Can you work these out from the model? Positions are in its coordinate system, mm. A direction names the side the tool comes from. Round coordinates to 2 decimals unless told otherwise and drop trailing zeros. Loops run counter-clockwise (first coordinate to the right, second up) from the corner with the lowest first, then second, coordinate; pieces in that order, holes last. Notation, with made-up numbers: (-21.75, 82) -> (-9.75, 82) arc R16 cw to (-9.75, 92) -> close; hole circle Ø3 at (87.25, 25). An arc over 180 degrees is marked (long way). Use a Markdown table: item, result.
from build123d import *

# Parameters (mm, degrees)
ESBO_O1_W                  = 50
ESBO_O1_H                  = 600
RESSALTO_EXTRUS_O1_DEPTH   = 200
ESBO_O1_W_2                = 47.772216991
RESSALTO_EXTRUS_O1_2_DEPTH = 200
RESSALTO_EXTRUS_O4_START   = -210
ESBO_O4_W                  = 600
ESBO_O4_H                  = 600
RESSALTO_EXTRUS_O4_DEPTH   = 10
ESBO_O5_W                  = 200
ESBO_O5_H                  = 190
CORTE_EXTRUS_O1_DEPTH      = 872.779788708
ESBO_O6_W                  = 200
ESBO_O6_H                  = 190
CORTE_EXTRUS_O2_DEPTH      = 600
FILETE2_R                  = 20
FILETE3_SIZE               = 20
FILETE4_SIZE               = 20
FILETE5_SIZE               = 20


with BuildPart() as part:
    # Esbo_o1 → Ressalto-extrus_o1 (new body)
    with BuildSketch(Plane(origin=(0, 0, 0), x_dir=(1, 0, 0), z_dir=(0, 1, 0))):
        with Locations((25, 300)):
            Rectangle(ESBO_O1_W, ESBO_O1_H)
    extrude(amount=RESSALTO_EXTRUS_O1_DEPTH)



with BuildPart() as body_2:
    # Esbo_o1 → Ressalto-extrus_o1 2 (new body)
    with BuildSketch(Plane(origin=(0, 0, 0), x_dir=(1, 0, 0), z_dir=(0, 1, 0))):
        with Locations((576.113891505, 300)):
            Rectangle(ESBO_O1_W_2, ESBO_O1_H)
    extrude(amount=RESSALTO_EXTRUS_O1_2_DEPTH)


with BuildPart() as part_1:
    add(part.part)

    add(body_2.part)  # Ressalto-extrus_o4 merges body 2
    # Esbo_o4 → Ressalto-extrus_o4 (add)
    with BuildSketch(Plane(origin=(0, 200, 0), x_dir=(1, 0, 0), z_dir=(0, 1, 0)).offset(RESSALTO_EXTRUS_O4_START)):
        with Locations((300, 300)):
            Rectangle(ESBO_O4_W, ESBO_O4_H)
    extrude(amount=RESSALTO_EXTRUS_O4_DEPTH)

    # Esbo_o5 → Corte-extrus_o1 (cut, through all)
    with BuildSketch(Plane(origin=(600, 0, 0), x_dir=(0, 0, -1), z_dir=(1, 0, 0))):
        with Locations((100, 105)):
            Rectangle(ESBO_O5_W, ESBO_O5_H)
    extrude(amount=-CORTE_EXTRUS_O1_DEPTH, mode=Mode.SUBTRACT)

    # Esbo_o6 → Corte-extrus_o2 (cut)
    with BuildSketch(Plane(origin=(600, 0, 0), x_dir=(0, 0, -1), z_dir=(1, 0, 0))):
        with Locations((500, 105)):
            Rectangle(ESBO_O6_W, ESBO_O6_H)
    extrude(amount=-CORTE_EXTRUS_O2_DEPTH, mode=Mode.SUBTRACT)

    # Filete2
    filete2_edges = [part_1.edges().sort_by_distance(p)[0] for p in [
        (576.113891505, 200, -200),
    ]]
    fillet(filete2_edges, radius=FILETE2_R)

    # Filete3
    # a fillet whose section is not a circle: 20 mm, written as the material it takes off along each edge
    with BuildSketch(Plane(origin=(650, 200, -400), x_dir=(0, 0, 1), z_dir=(-1, 0, 0))) as filete3_piece_1:
        with BuildLine():
            add(Edge.make_bspline([(FILETE3_SIZE, 0), (FILETE3_SIZE * 0.831801948466, 0), (FILETE3_SIZE * 0.663603896932, 0), (FILETE3_SIZE * 0.292893218813, -FILETE3_SIZE * 0.0716919198361), (FILETE3_SIZE * 0.0716919198361, -FILETE3_SIZE * 0.292893218813), (0, -FILETE3_SIZE * 0.663603896932), (0, -FILETE3_SIZE * 0.831801948466), (0, -FILETE3_SIZE)], knots=[0, 0, 0, 0, 0, 0, 0.5, 0.5, 1, 1, 1, 1, 1, 1], degree=5))
            Line((0, -FILETE3_SIZE), (0, 0))
            Line((0, 0), (FILETE3_SIZE, 0))
        make_face()
    extrude(amount=147.772216991, mode=Mode.SUBTRACT)

    # Filete4
    # a fillet whose section is not a circle: 20 mm, written as the material it takes off along each edge
    with BuildSketch(Plane(origin=(100, 200, -200), x_dir=(0, -1, 0), z_dir=(-1, 0, 0))) as filete4_piece_1:
        with BuildLine():
            add(Edge.make_bspline([(FILETE4_SIZE, 0), (FILETE4_SIZE * 0.831801948466, 0), (FILETE4_SIZE * 0.663603896932, 0), (FILETE4_SIZE * 0.292893218813, -FILETE4_SIZE * 0.0716919198361), (FILETE4_SIZE * 0.0716919198361, -FILETE4_SIZE * 0.292893218813), (0, -FILETE4_SIZE * 0.663603896932), (0, -FILETE4_SIZE * 0.831801948466), (0, -FILETE4_SIZE)], knots=[0, 0, 0, 0, 0, 0, 0.5, 0.5, 1, 1, 1, 1, 1, 1], degree=5))
            Line((0, -FILETE4_SIZE), (0, 0))
            Line((0, 0), (FILETE4_SIZE, 0))
        make_face()
    extrude(amount=150, mode=Mode.SUBTRACT)

    # Filete5
    # a fillet whose section is not a circle: 20 mm, written as the material it takes off along each edge
    with BuildSketch(Plane(origin=(100, 200, -400), x_dir=(0, 0, 1), z_dir=(-1, 0, 0))) as filete5_piece_1:
        with BuildLine():
            add(Edge.make_bspline([(FILETE5_SIZE, 0), (FILETE5_SIZE * 0.831801948466, 0), (FILETE5_SIZE * 0.663603896932, 0), (FILETE5_SIZE * 0.292893218813, -FILETE5_SIZE * 0.0716919198361), (FILETE5_SIZE * 0.0716919198361, -FILETE5_SIZE * 0.292893218813), (0, -FILETE5_SIZE * 0.663603896932), (0, -FILETE5_SIZE * 0.831801948466), (0, -FILETE5_SIZE)], knots=[0, 0, 0, 0, 0, 0, 0.5, 0.5, 1, 1, 1, 1, 1, 1], degree=5))
            Line((0, -FILETE5_SIZE), (0, 0))
            Line((0, 0), (FILETE5_SIZE, 0))
        make_face()
    extrude(amount=150, mode=Mode.SUBTRACT)


solid = part_1.part
1. I want a section at B-B (z = -491). Please give me the cut outline in (x, y), plus the area to 3 significant figures.
Answer sheet:
| item | result |
|---|---|
| outline | (0, -10) -> (600, -10) -> (600, 10) -> (552.23, 10) -> (552.23, 0) -> (50, 0) -> (50, 10) -> (0, 10) -> close |
| area | 6,980 mm² |
2. Will these pins go through, and if not, where does the flat tip stop? pin 1 Ø14.5 at (x, y) = (570, 114.5) entering from -Z; pin 2 Ø3 at (x, z) = (424.5, -315) entering from +Y; pin 3 Ø14.5 at (x, z) = (582.5, -52.5) entering from +Y.
Answer sheet:
| item | result |
|---|---|
| pin 1 | stops at z = -400 |
| pin 2 | stops at y = 0 |
| pin 3 | stops at y = 10 |
3. I want a section at C-C (x = 522). Please give me the cut outline in (y, z), plus the area to 3 significant figures.
Answer sheet:
| item | result |
|---|---|
| outline | (-10, -600) -> (0, -600) -> (0, 0) -> (-10, 0) -> close |
| area | 6,000 mm² |
4. I want a section at D-D (z = -285.5). Please give me the cut outline in (x, y).
Answer sheet:
| item | result |
|---|---|
| outline | (0, -10) -> (600, -10) -> (600, 200) -> (552.23, 200) -> (552.23, 0) -> (50, 0) -> (50, 200) -> (0, 200) -> close |
5. Which directions (+Z, -Z, +X, -X, +Y, -Y) give clear straight access to the entire face, cutting with the end or side of a thin tool? Please do faces 1 (the flat face through (25, 10, -99)), 2 (the flat face through (576, 94, -400)), 3 (the flat face through (298, 0, -304)).
Answer sheet:
| item | result |
|---|---|
| face 1 | +Z, +X, -X, +Y |
| face 2 | -Z, +X, -X, +Y |
| face 3 | +Z, -Z, +Y |
6. I need wall thicknesses on line 1 (X direction, y = 124, z = -204.5); line 2 (Y direction, x = 443, z = -315); line 3 (Y direction, x = 562.5, z = -570.5). Which ranges of each line are inside material? Lowest first, please.
Answer sheet:
| item | result |
|---|---|
| line 1 | x = 0 to 50, 552.23 to 600 |
| line 2 | y = -10 to 0 |
| line 3 | y = -10 to 10 |
7. I want a section at A-A (y = 169). Please give me the cut outline in (x, z).
Answer sheet:
| item | result |
|---|---|
| outline | (0, -400) -> (50, -400) -> (50, -200) -> (0, -200) -> close; (552.23, -400) -> (600, -400) -> (600, -200) -> (552.23, -200) -> close |
8. If we mould it in two halves opening along X, with no side actions, what happens to faces 4 (the flat face through (576, 94, -200)), 5 (the flat face through (552.228, 76, -296)), 6 (the flat face through (600, 70, -296))? For each: +X half, -X half, draft (parallel to the pull), parting line (faces both ways), or undercut.
Answer sheet:
| item | result |
|---|---|
| face 4 | draft |
| face 5 | undercut |
| face 6 | +X half |
